Autodesk Inventor part; units mm, degrees
ref_plane "YZ Plane" through (0, 0, 0) normal (1, 0, 0) x (0, 1, 0)
ref_plane "XZ Plane" through (0, 0, 0) normal (0, 1, 0) x (-1, 0, 0)
ref_plane "XY Plane" through (0, 0, 0) normal (0, 0, 1) x (1, 0, 0)
sketch "スケッチ1" plane through (0, 0, 0) normal (0, 0, 1) x (1, 0, 0)
  circle A0 centre (-26.15, 0) radius 1.1
  circle A1 centre (-20.55, 3) radius 0.4
  circle A2 centre (-18.85, 4.5) radius 0.4 construction
  circle A3 centre (-20.55, 1) radius 0.4
  circle A4 centre (-20.55, -1) radius 0.4
  circle A5 centre (-20.55, -3) radius 0.4
  circle A6 centre (-14.55, 3) radius 0.4
  circle A7 centre (-12.85, 4.5) radius 0.4 construction
  circle A8 centre (-14.55, 1) radius 0.4
  circle A9 centre (-14.55, -1) radius 0.4
  circle A10 centre (-14.55, -3) radius 0.4
  circle A11 centre (-8.55, 3) radius 0.4
  circle A12 centre (-6.85, 4.5) radius 0.4 construction
  circle A13 centre (-8.55, 1) radius 0.4
  circle A14 centre (-8.55, -1) radius 0.4
  circle A15 centre (-8.55, -3) radius 0.4
  circle A16 centre (-2.55, 3) radius 0.4
  circle A17 centre (-0.85, 4.5) radius 0.4 construction
  circle A18 centre (-2.55, 1) radius 0.4
  circle A19 centre (-2.55, -1) radius 0.4
  circle A20 centre (-2.55, -3) radius 0.4
  circle A21 centre (3.45, 3) radius 0.4
  circle A22 centre (5.15, 4.5) radius 0.4 construction
  circle A23 centre (3.45, 1) radius 0.4
  circle A24 centre (3.45, -1) radius 0.4
  circle A25 centre (3.45, -3) radius 0.4
  circle A26 centre (9.45, 3) radius 0.4
  circle A27 centre (11.15, 4.5) radius 0.4 construction
  circle A28 centre (9.45, 1) radius 0.4
  circle A29 centre (9.45, -1) radius 0.4
  circle A30 centre (9.45, -3) radius 0.4
  circle A31 centre (15.45, 3) radius 0.4
  circle A32 centre (17.15, 4.5) radius 0.4 construction
  circle A33 centre (15.45, 1) radius 0.4
  circle A34 centre (15.45, -1) radius 0.4
  circle A35 centre (15.45, -3) radius 0.4
  circle A36 centre (21.45, 3) radius 0.4
  circle A37 centre (23.15, 4.5) radius 0.4 construction
  circle A38 centre (21.45, 1) radius 0.4
  circle A39 centre (21.45, -1) radius 0.4
  circle A40 centre (21.45, -3) radius 0.4
  line L0 (-26.1134, -4.9138) -> (-27.9707, -0.8276)
  arc A41 (-27.9707, 0.8276) -> (-27.9707, -0.8276) centre (-26.15, 0) ccw
  line L1 (-27.9707, 0.8276) -> (-26.1134, 4.9138)
  arc A42 (-25.203, 5.5) -> (-26.1134, 4.9138) centre (-25.203, 4.5) ccw
  line L2 (-25.203, 5.5) -> (25.203, 5.5)
  arc A43 (26.1134, 4.9138) -> (25.203, 5.5) centre (25.203, 4.5) ccw
  line L3 (26.1134, 4.9138) -> (27.9707, 0.8276)
  arc A44 (27.9707, -0.8276) -> (27.9707, 0.8276) centre (26.15, 0) ccw
  line L4 (27.9707, -0.8276) -> (26.1134, -4.9138)
  arc A45 (25.203, -5.5) -> (26.1134, -4.9138) centre (25.203, -4.5) ccw
  line L5 (25.203, -5.5) -> (-25.203, -5.5)
  arc A46 (-26.1134, -4.9138) -> (-25.203, -5.5) centre (-25.203, -4.5) ccw
  circle A47 centre (26.15, 0) radius 1.1
  line L6 (-26.15, 0) -> (26.15, 0) construction
  line L7 (0, 0) -> (0, 14.1732) construction
  circle A48 centre (-18.85, -4.5) radius 0.4
  circle A49 centre (-12.85, -4.5) radius 0.4
  circle A50 centre (-6.85, -4.5) radius 0.4
  circle A51 centre (-0.85, -4.5) radius 0.4
  circle A52 centre (5.15, -4.5) radius 0.4
  circle A53 centre (11.15, -4.5) radius 0.4
  circle A54 centre (17.15, -4.5) radius 0.4
  circle A55 centre (23.15, -4.5) radius 0.4
extrude "押し出し1" add sketch "スケッチ1" along normal blind 1.6
properties part number "IMUTrackerBase_8port_hub_pcb"
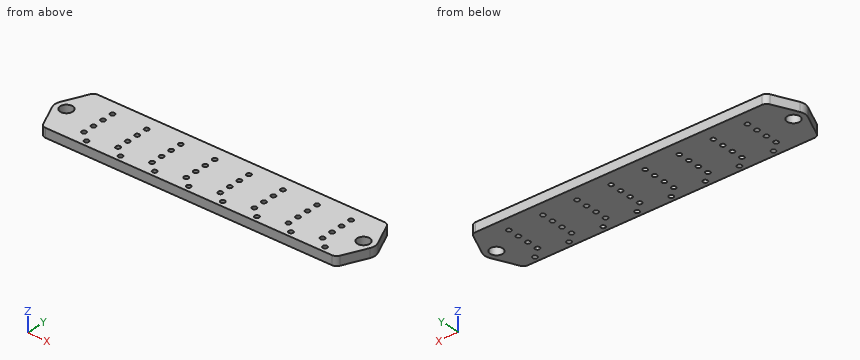
The listing builds one solid part. Answer for the finished solid, in the listing's coordinates (mm). Coordinates: 2 decimals unless noted, no trailing zeros. Answer in a Markdown table with one row per item. Add a question column.
Item 1: Find section A-A (z = 1.25). State how many separate pieces and enclosed holes the cut face has, then the cut area to 3 significant figures.
Item 2: Find the intervals of material crossed by L1, parallel to Y at x = -20.55, z = 0.55; L2, parallel to Y at x = -13, z = 0.8; L3, parallel to X at y = -4, z = 0.25, in increasing order. Write a range as from..to.
Item 3: This flat-tipped pin is pushed along its axis until it touches: P1, Ø3.5, axis at x = 26.15, y = 0, coming from the +Z side. Where does it stop, or does it pass through?
Result set:
| question | item | result |
|---|---|---|
| 1 | separate pieces | 1 |
| 1 | enclosed holes | 42 |
| 1 | area | 568 mm² |
| 2 | L1 | y = -5.5..-3.4, -2.6..-1.4, -0.6..0.6, 1.4..2.6, 3.4..5.5 |
| 2 | L2 | y = -5.5..-4.87, -4.13..5.5 |
| 2 | L3 | x = -26.53..26.53 |
| 3 | P1 | stops at z = 1.6 |
